Verification items for the finished model (mm, model axes). Round coordinates to 2 decimals unless told otherwise and drop trailing zeros. Order: outer loops, then holes, each group sorted by start corner. A loop starts at its lowest first (then second) coordinate and runs counter-clockwise, first axis right, second up. Notation, with made-up numbers: M 58,-10.75 L 70,-10.75 A12 ccw 70,3.25 Z; hole C -3.75,80 d8. An arc over 180 degrees is marked long. Use one line per item in the form item = value. Start each with the question number.
Item 1: Cross-section at B-B on x = -22.5. Enter the section's corners in (y, z), then the cut area to 3 significant figures.
Item 2: Go/stop test with flat-tipped pins: pin 1 Ø3 at (x, z) = (-67.5, 14) entering from +Y; pin 2 Ø1.2 at (x, z) = (-68.5, -34.5) entering from -Y. Record where each tip stops, or that it passes through.
Item 3: Cross-section at D-D on z = 1. Enter the section's corners in (x, y).
Item 4: Cross-section at A-A on x = 12.5. Enter the section's corners in (y, z), then the cut area to 3 significant figures.
Item 5: Thickness scan on probe 1 along X at (y, z) = (4.25, 23.2); probe 2 along X at (y, z) = (5, 40); probe 3 along Z at (x, y) = (-73, 3.5). Record the ranges inside material, lowest first. Write a range as [from, to].
Item 6: Release check for a two-part mould opening along Z. For faces 1 (the cylindrical face through (28.26, 3.3, 24.82)), 2 (the flat face through (85, 3, 1)) record: +Z half, -Z half, draft (parallel to the pull), parting line (faces both ways), or undercut.
Item 7: Cross-section at C-C on z = -35.15. Count the separate pieces of the cut face and the enclosed holes in it, then the cut area to 3 significant figures.
from build123d import *

# Parameters (mm, degrees)
SKETCH_1_W           = 100
SKETCH_1_H           = 100
EXTRUDE_1_DEPTH      = 6.5
SKETCH_2_W           = 5
SKETCH_2_H           = 100
EXTRUDE_2_DEPTH      = 75
SKETCH_3_R           = 2.25
CUT_EXTRUDE_1_DEPTH  = 85
SKETCH_4_W           = 40
SKETCH_4_H           = 41.42
CUT_EXTRUDE_2_DEPTH  = 85
CHAMFER_1_SIZE       = 10
SKETCH_5_W           = 10
SKETCH_5_H           = 30
CUT_EXTRUDE_3_DEPTH  = 85
SKETCH_11_R          = 1.7
CUT_EXTRUDE_5_DEPTH  = 10
SKETCH_12_R          = 1.7
CUT_EXTRUDE_6_DEPTH  = 25
SKETCH_13_R          = 2.3
SKETCH_13_R_2        = 15
CUT_EXTRUDE_9_DEPTH  = 105
SKETCH_14_W          = 15
SKETCH_14_H          = 41.42
CUT_EXTRUDE_10_DEPTH = 83
SKETCH_15_W          = 38.97610678
SKETCH_15_H          = 41.42
CUT_EXTRUDE_11_DEPTH = 83
SKETCH_16_R          = 1.7
CUT_EXTRUDE_12_DEPTH = 83
SKETCH_17_R          = 2.15
CUT_EXTRUDE_13_DEPTH = 83
CHAMFER_2_SIZE       = 8
SKETCH_18_W          = 143.568344584
SKETCH_18_H          = 92.865991502
CUT_EXTRUDE_14_DEPTH = 55
SKETCH_19_W          = 35
SKETCH_19_H          = 100
EXTRUDE_3_DEPTH      = 6.5
SKETCH_21_R          = 10.75
CUT_EXTRUDE_16_DEPTH = 10
SKETCH_20_R          = 2.1
CUT_EXTRUDE_15_DEPTH = 7.5
SKETCH_23_W          = 20.3
SKETCH_23_H          = 40.4
CUT_EXTRUDE_17_DEPTH = 20
SKETCH_24_W          = 2.5
SKETCH_24_H          = 18
CUT_EXTRUDE_18_DEPTH = 2.4
SKETCH_25_R          = 1.6
CUT_EXTRUDE_19_DEPTH = 10
SKETCH_26_W          = 8
SKETCH_26_H          = 20
CUT_EXTRUDE_20_DEPTH = 23


with BuildPart() as part:
    # 草图1 → 凸台-拉伸1 (new body)
    with BuildSketch(Plane(origin=(0, 0, 0), x_dir=(1, 0, 0), z_dir=(0, 1, 0))):
        Rectangle(SKETCH_1_W, SKETCH_1_H)
    extrude(amount=EXTRUDE_1_DEPTH)

    # 草图2 → 凸台-拉伸2 (add)
    with BuildSketch(Plane.XZ):
        with Locations((-34.5, 0)):
            Rectangle(SKETCH_2_W, SKETCH_2_H)
        with Locations((34.5, 0)):
            Rectangle(SKETCH_2_W, SKETCH_2_H)
    extrude(amount=EXTRUDE_2_DEPTH)

    # 草图3 → 切除-拉伸1 (cut)
    with BuildSketch(Plane.ZY.offset(37)):
        with Locations((-4.925, -12)):
            Circle(SKETCH_3_R)
        with Locations((4.925, -12)):
            Circle(SKETCH_3_R)
        with Locations((-4.925, -61.42)):
            Circle(SKETCH_3_R)
        with Locations((4.925, -61.42)):
            Circle(SKETCH_3_R)
        with Locations((14.773492699, -12.172312361)):
            Circle(SKETCH_3_R)
        with Locations((14.773492699, -61.247687639)):
            Circle(SKETCH_3_R)
        with Locations((-14.773492699, -61.247687639)):
            Circle(SKETCH_3_R)
        with Locations((-14.773492699, -12.172312361)):
            Circle(SKETCH_3_R)
    extrude(amount=-CUT_EXTRUDE_1_DEPTH, mode=Mode.SUBTRACT)

    # 草图4 → 切除-拉伸2 (cut)
    with BuildSketch(Plane.ZY.offset(37)):
        with Locations((0, -36.71)):
            Rectangle(SKETCH_4_W, SKETCH_4_H)
    extrude(amount=-CUT_EXTRUDE_2_DEPTH, mode=Mode.SUBTRACT)

    # 倒角1
    chamfer_1_edges = [part.edges().sort_by_distance(p)[0] for p in [
        (-34.5, -75, 50),
        (-34.5, -75, -50),
        (34.5, -75, 50),
        (34.5, -75, -50),
    ]]
    chamfer(chamfer_1_edges, length=CHAMFER_1_SIZE)

    # 草图5 → 切除-拉伸3 (cut)
    with BuildSketch(Plane(origin=(0, 6.5, 0), x_dir=(1, 0, 0), z_dir=(0, 1, 0))):
        with Locations((-25, 0)):
            Rectangle(SKETCH_5_W, SKETCH_5_H)
        with Locations((25, 0)):
            Rectangle(SKETCH_5_W, SKETCH_5_H)
    extrude(amount=-CUT_EXTRUDE_3_DEPTH, mode=Mode.SUBTRACT)

    # 草图11 → 切除-拉伸5 (cut)
    with BuildSketch(Plane.XZ):
        with Locations(Location((-44, 38, 0), (0, 0, 270))):
            Circle(SKETCH_11_R)
        with Locations(Location((-44, 26, 0), (0, 0, 270))):
            Circle(SKETCH_11_R)
        with Locations(Location((-44, 14, 0), (0, 0, 270))):
            Circle(SKETCH_11_R)
        with Locations(Location((44, 14, 0), (0, 0, 270))):
            Circle(SKETCH_11_R)
        with Locations(Location((44, 26, 0), (0, 0, 270))):
            Circle(SKETCH_11_R)
        with Locations(Location((44, 38, 0), (0, 0, 270))):
            Circle(SKETCH_11_R)
        with Locations(Location((44, -38, 0), (0, 0, 270))):
            Circle(SKETCH_11_R)
        with Locations(Location((44, -26, 0), (0, 0, 270))):
            Circle(SKETCH_11_R)
        with Locations(Location((44, -14, 0), (0, 0, 270))):
            Circle(SKETCH_11_R)
        with Locations(Location((-44, -14, 0), (0, 0, 270))):
            Circle(SKETCH_11_R)
        with Locations(Location((-44, -26, 0), (0, 0, 270))):
            Circle(SKETCH_11_R)
        with Locations(Location((-44, -38, 0), (0, 0, 270))):
            Circle(SKETCH_11_R)
    extrude(amount=-CUT_EXTRUDE_5_DEPTH, mode=Mode.SUBTRACT)

    # 草图12 → 切除-拉伸6 (cut)
    with BuildSketch(Plane(origin=(0, 6.5, 0), x_dir=(1, 0, 0), z_dir=(0, 1, 0))):
        with Locations(Location((-27.75, 42, 0), (0, 0, 270))):
            Circle(SKETCH_12_R)
        with Locations(Location((-27.75, 23.2, 0), (0, 0, 270))):
            Circle(SKETCH_12_R)
        with Locations(Location((27.75, 23.2, 0), (0, 0, 90))):
            Circle(SKETCH_12_R)
        with Locations(Location((27.75, 42, 0), (0, 0, 90))):
            Circle(SKETCH_12_R)
        with Locations(Location((27.75, -42, 0), (0, 0, 270))):
            Circle(SKETCH_12_R)
        with Locations(Location((27.75, -23.2, 0), (0, 0, 270))):
            Circle(SKETCH_12_R)
        with Locations(Location((-27.75, -23.2, 0), (0, 0, 90))):
            Circle(SKETCH_12_R)
        with Locations(Location((-27.75, -42, 0), (0, 0, 90))):
            Circle(SKETCH_12_R)
    extrude(amount=-CUT_EXTRUDE_6_DEPTH, mode=Mode.SUBTRACT)

    # 草图13 → 切除-拉伸9 (cut)
    with BuildSketch(Plane.ZY.offset(37)):
        with Locations((46, -16)):
            Circle(SKETCH_13_R)
        with Locations((46, -51)):
            Circle(SKETCH_13_R)
        with Locations((46, -33.5)):
            Circle(SKETCH_13_R_2)
    extrude(amount=-CUT_EXTRUDE_9_DEPTH, mode=Mode.SUBTRACT)

    # 草图14 → 切除-拉伸10 (cut)
    with BuildSketch(Plane.ZY.offset(37)):
        with Locations((-27.5, -36.71)):
            Rectangle(SKETCH_14_W, SKETCH_14_H)
    extrude(amount=-CUT_EXTRUDE_10_DEPTH, mode=Mode.SUBTRACT)

    # 草图15 → 切除-拉伸11 (cut)
    with BuildSketch(Plane.ZY.offset(37)):
        with Locations((-35, -36.71)):
            Rectangle(SKETCH_15_W, SKETCH_15_H)
    extrude(amount=-CUT_EXTRUDE_11_DEPTH, mode=Mode.SUBTRACT)

    # 草图16 → 切除-拉伸12 (cut)
    with BuildSketch(Plane(origin=(0, 6.5, 0), x_dir=(1, 0, 0), z_dir=(0, 1, 0))):
        with Locations(Location((-12.5, 15, 0), (0, 0, 270))):
            Circle(SKETCH_16_R)
        with Locations(Location((12.5, 15, 0), (0, 0, 90))):
            Circle(SKETCH_16_R)
        with Locations(Location((12.5, -15, 0), (0, 0, 270))):
            Circle(SKETCH_16_R)
        with Locations(Location((-12.5, -15, 0), (0, 0, 90))):
            Circle(SKETCH_16_R)
    extrude(amount=-CUT_EXTRUDE_12_DEPTH, mode=Mode.SUBTRACT)

    # 草图17 → 切除-拉伸13 (cut)
    with BuildSketch(Plane.ZY.offset(37)):
        with Locations((-24.623492699, -12.172312361)):
            Circle(SKETCH_17_R)
        with Locations((-24.625, -61.42)):
            Circle(SKETCH_17_R)
        with Locations((-39.622497813, -11.999553542)):
            Circle(SKETCH_17_R)
        with Locations((-39.622497813, -61.420446458)):
            Circle(SKETCH_17_R)
    extrude(amount=-CUT_EXTRUDE_13_DEPTH, mode=Mode.SUBTRACT)

    # 倒角2
    chamfer_2_edges = [part.edges().sort_by_distance(p)[0] for p in [
        (34.5, -16, -50),
        (-34.5, -16, -50),
    ]]
    chamfer(chamfer_2_edges, length=CHAMFER_2_SIZE)

    # 草图18 → 切除-拉伸14 (cut, symmetric)
    with BuildSketch(Plane(origin=(0, 0, 0), x_dir=(0, 0, -1), z_dir=(1, 0, 0))):
        with Locations((21.784172292, -46.432995751)):
            Rectangle(SKETCH_18_W, SKETCH_18_H)
    extrude(amount=CUT_EXTRUDE_14_DEPTH, both=True, mode=Mode.SUBTRACT)

    # 草图19 → 凸台-拉伸3 (add)
    with BuildSketch(Plane(origin=(0, 0, 0), x_dir=(1, 0, 0), z_dir=(0, 1, 0))):
        with Locations((-67.5, 0)):
            Rectangle(SKETCH_19_W, SKETCH_19_H)
        with Locations((67.5, 0)):
            Rectangle(SKETCH_19_W, SKETCH_19_H)
    extrude(amount=EXTRUDE_3_DEPTH)

    # 草图21 → 切除-拉伸16 (cut)
    with BuildSketch(Plane.XZ):
        with Locations(Location((-68, 0, 0), (0, 0, 270))):
            Circle(SKETCH_21_R)
        with Locations(Location((68, 0, 0), (0, 0, 270))):
            Circle(SKETCH_21_R)
    extrude(amount=-CUT_EXTRUDE_16_DEPTH, mode=Mode.SUBTRACT)

    # 草图20 → 切除-拉伸15 (cut, symmetric)
    with BuildSketch(Plane(origin=(0, 6.5, 0), x_dir=(1, 0, 0), z_dir=(0, 1, 0))):
        with Locations(Location((-63, -14.35, 0), (0, 0, 90))):
            Circle(SKETCH_20_R)
        with Locations(Location((-73, -14.35, 0), (0, 0, 90))):
            Circle(SKETCH_20_R)
        with Locations(Location((-73, 35.15, 0), (0, 0, 90))):
            Circle(SKETCH_20_R)
        with Locations(Location((-63, 35.15, 0), (0, 0, 90))):
            Circle(SKETCH_20_R)
        with Locations(Location((63, 35.15, 0), (0, 0, 90))):
            Circle(SKETCH_20_R)
        with Locations(Location((73, 35.15, 0), (0, 0, 90))):
            Circle(SKETCH_20_R)
        with Locations(Location((73, -14.35, 0), (0, 0, 90))):
            Circle(SKETCH_20_R)
        with Locations(Location((63, -14.35, 0), (0, 0, 90))):
            Circle(SKETCH_20_R)
    extrude(amount=CUT_EXTRUDE_15_DEPTH, both=True, mode=Mode.SUBTRACT)

    # 草图23 → 切除-拉伸17 (cut)
    with BuildSketch(Plane(origin=(0, 6.5, 0), x_dir=(1, 0, 0), z_dir=(0, 1, 0))):
        with Locations((-68, 10.4)):
            Rectangle(SKETCH_23_W, SKETCH_23_H)
        with Locations((68, 10.4)):
            Rectangle(SKETCH_23_W, SKETCH_23_H)
    extrude(amount=-CUT_EXTRUDE_17_DEPTH, mode=Mode.SUBTRACT)

    # 草图24 → 切除-拉伸18 (cut)
    with BuildSketch(Plane(origin=(0, 6.5, 0), x_dir=(1, 0, 0), z_dir=(0, 1, 0))):
        with Locations((-68, 30.6)):
            Rectangle(SKETCH_24_W, SKETCH_24_H)
        with Locations((68, 30.6)):
            Rectangle(SKETCH_24_W, SKETCH_24_H)
        with Locations((68, -9.8)):
            Rectangle(SKETCH_24_W, SKETCH_24_H)
        with Locations((-68, -9.8)):
            Rectangle(SKETCH_24_W, SKETCH_24_H)
    cut_extrude_18 = extrude(amount=-CUT_EXTRUDE_18_DEPTH, mode=Mode.SUBTRACT)

    # 草图25 → 切除-拉伸19 (cut)
    with BuildSketch(Plane(origin=(0, 6.5, 0), x_dir=(1, 0, 0), z_dir=(0, 1, 0))):
        with Locations(Location((-79, 40, 0), (0, 0, 270))):
            Circle(SKETCH_25_R)
        with Locations((-87.320502943, 27.519245585)):
            Circle(SKETCH_25_R)
        with Locations((87.320502943, 27.519245585)):
            Circle(SKETCH_25_R)
        with Locations(Location((79, 40, 0), (0, 0, 90))):
            Circle(SKETCH_25_R)
        with Locations(Location((79, -40, 0), (0, 0, 270))):
            Circle(SKETCH_25_R)
        with Locations((87.320502943, -27.519245585)):
            Circle(SKETCH_25_R)
        with Locations((-87.320502943, -27.519245585)):
            Circle(SKETCH_25_R)
        with Locations(Location((-79, -40, 0), (0, 0, 90))):
            Circle(SKETCH_25_R)
    extrude(amount=-CUT_EXTRUDE_19_DEPTH, mode=Mode.SUBTRACT)

    # 草图26 → 切除-拉伸20 (cut)
    with BuildSketch(Plane(origin=(0, 6.5, 0), x_dir=(1, 0, 0), z_dir=(0, 1, 0))):
        with Locations((-46, -32)):
            Rectangle(SKETCH_26_W, SKETCH_26_H)
        with Locations((46, -32)):
            Rectangle(SKETCH_26_W, SKETCH_26_H)
        with Locations((46, 32)):
            Rectangle(SKETCH_26_W, SKETCH_26_H)
        with Locations((-46, 32)):
            Rectangle(SKETCH_26_W, SKETCH_26_H)
    extrude(amount=-CUT_EXTRUDE_20_DEPTH, mode=Mode.SUBTRACT)

    # 镜向1: 切除-拉伸18 across plane
    add(cut_extrude_18.mirror(Plane.ZX.offset(3.25)), mode=Mode.SUBTRACT)


solid = part.part
Output values:
q1.outline = M 0,-50 L 6.5,-50 L 6.5,-15 L 0,-15 Z; M 0,15 L 6.5,15 L 6.5,50 L 0,50 Z
q1.area = 455 mm2
q2.pin_1 = 6.5
q2.pin_2 = 2.4
q3.outline = M -85,0 L -78.7,0 L -78.7,6.5 L -85,6.5 Z; M -57.3,0 L -30,0 L -30,6.5 L -57.3,6.5 Z; M -20,0 L 20,0 L 20,6.5 L -20,6.5 Z; M 30,0 L 57.3,0 L 57.3,6.5 L 30,6.5 Z; M 78.7,0 L 85,0 L 85,6.5 L 78.7,6.5 Z
q4.outline = M 0,-50 L 6.5,-50 L 6.5,-16.7 L 0,-16.7 Z; M 0,-13.3 L 6.5,-13.3 L 6.5,13.3 L 0,13.3 Z; M 0,16.7 L 6.5,16.7 L 6.5,50 L 0,50 Z
q4.area = 606 mm2
q5.probe_1 = [-85, -50], [-42, -29.45], [-26.05, 26.05], [29.45, 42], [50, 85]
q5.probe_2 = [-85, -80.6], [-77.4, -50], [-42, 42], [50, 77.4], [80.6, 85]
q5.probe_3 = [-50, -37.25], [-33.05, -30.6], [9.8, 12.25], [16.45, 50]
q6.face_1 = undercut
q6.face_2 = draft
q7.separate_pieces = 7
q7.enclosed_holes = 0
q7.area = 868 mm2
